Could you check a few things on this drawing? It's one solid part, dimensions in mm from its lowest x, y, z. A direction names the side the tool comes from. Round coordinates to 2 decimals unless told otherwise and drop trailing zeros. Order: outer loops, then holes, each group sorted by start corner. A loop starts at its lowest first (then second) coordinate and runs counter-clockwise, first axis right, second up. Notation, with made-up numbers: (40.5, 44) - (90.5, 44) arc R16 ccw to (90.5, 69) - close; hole circle Ø8 at (81.5, 68.25). An arc over 180 degrees is marked (long way). Use one line per item in the form item = value.
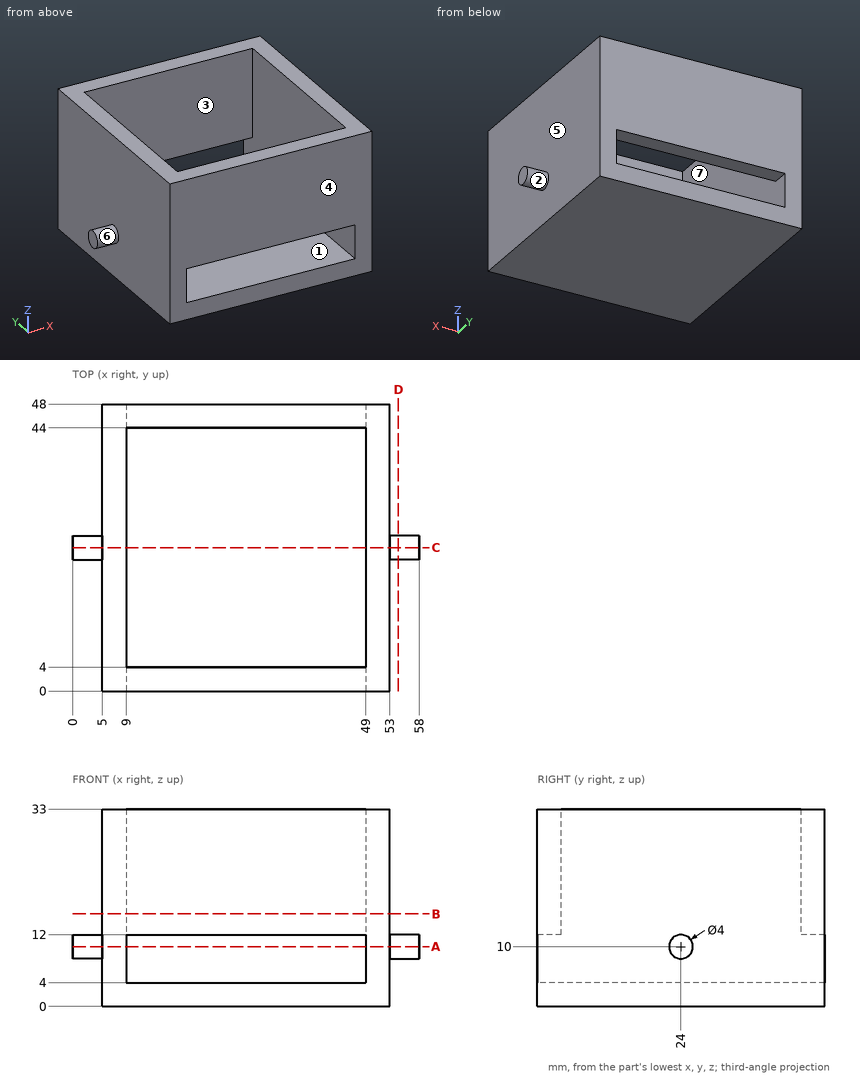
Item 1: Imagine slicing it at C-C on y = 24. Please give me the cut outline in (x, z), plus the area to 3 significant figures.
Found:
outline = (0, 8) - (5, 8) - (5, 0) - (53, 0) - (53, 8) - (58, 8) - (58, 12) - (53, 12) - (53, 33) - (49, 33) - (49, 4) - (9, 4) - (9, 33) - (5, 33) - (5, 12) - (0, 12) - close
area = 464 mm2
Item 2: If we mould it in two halves opening along Y, with no side actions, what happens to the marked faces 4, 5, 6 and 7? For each: released by +Y, released by -Y, zero draft, split by the parting line, or undercut.
Found:
face_4 = released by -Y
face_5 = zero draft
face_6 = split by the parting line
face_7 = undercut
Item 3: Imagine slicing it at A-A on z = 10. Please give me the cut outline in (x, y), plus the area to 3 significant figures.
Found:
outline = (0, 22) - (5, 22) - (5, 0) - (9, 0) - (9, 48) - (5, 48) - (5, 26) - (0, 26) - close; (49, 0) - (53, 0) - (53, 22) - (58, 22) - (58, 26) - (53, 26) - (53, 48) - (49, 48) - close
area = 424 mm2
Item 4: Imagine slicing it at B-B on z = 15.5. Please give me the cut outline in (x, y).
Found:
outline = (5, 0) - (53, 0) - (53, 48) - (5, 48) - close; hole (9, 4) - (49, 4) - (49, 44) - (9, 44) - close
Item 5: For the marked faces 1, 2 and 3, which set-ups out of +Z, -Z, +X, -X, +Y, -Y let a thin tool reach every point of the face, with its end or its side?
Found:
face_1 = +Y, -Y
face_2 = +X
face_3 = +Z
Item 6: I need wall thicknesses on L1, parallel to X at y = 22.5, z = 19; L2, parallel to Y at x = 29, z = 19; L3, parallel to X at y = 9, z = 3. Which ranges of each line are inside material? Lowest first, please.
Found:
L1 = 5 to 9, 49 to 53
L2 = 0 to 4, 44 to 48
L3 = 5 to 53
Item 7: Will these pins go through, and if not, where does the flat tip stop? P1, Ø8, axis at x = 42, z = 6, coming from the +Y side; P2, Ø3, axis at y = 16.5, z = 21, coming from the -X side; P3, Ø6, axis at x = 29.5, y = 14.5, coming from the +Z side.
Found:
P1 = 48
P2 = 5
P3 = 4
Item 8: Imagine slicing it at D-D on x = 54.5. Please give me the cut outline in (y, z).
Found:
outline = circle Ø4 at (24, 10)
